Source: CAD feature listing. Evaluate the final solid. Frame: model axes, mm. Face numbers are marked on the shaded views. A direction names the side the tool comes from. Give positions to 0.01 mm unless a question says otherwise; leave off trailing zeros. Order: outer loops, then holes, each group sorted by start corner. A loop starts at its lowest first (then second) coordinate and runs counter-clockwise, first axis right, second up. Notation, with made-up numbers: (27.5, 36) -> (43.5, 36) arc R11 ccw to (43.5, 47) -> close; hole circle Ø4 at (72, 30). An arc over 180 degrees is marked (long way). Use one line per item in the form item = value. Start each with the question number.
from build123d import *

# Parameters (mm, degrees)
F0_R      = 76.2
F1_DEPTH  = 25.4
F2_R      = 5.08
F1_FACE_R = 71.12
F3_DEPTH  = 6.35
F4_R      = 3.175
F5_DEPTH  = 25.4
F6_R      = 59.059026
F7_DEPTH  = 21.59
F9_DEPTH  = 22.86
F11_DEPTH = 23.368
F13_DEPTH = 25.4


with BuildPart() as f1:
    # F0 (on Front) → F1 (new body)
    with BuildSketch(Plane.XZ):
        Circle(F0_R)
    extrude(amount=F1_DEPTH)

    # F2
    f2_edges = [f1.edges().sort_by_distance(p)[0] for p in [
        (76.2, -12.7, 0),
        (-76.2, 0, 0),
        (-76.2, -25.4, 0),
    ]]
    fillet(f2_edges, radius=F2_R)

    # F1_face (on face) → F3 (cut)
    with BuildSketch(Plane.XZ.offset(25.4)):
        Circle(F1_FACE_R)
    extrude(amount=-F3_DEPTH, mode=Mode.SUBTRACT)

    # F4 (on Front) → F5 (cut)
    with BuildSketch(Plane.XZ):
        with Locations((0, 66.04)):
            Circle(F4_R)
    extrude(amount=F5_DEPTH, mode=Mode.SUBTRACT)

    # F6 (on Front) → F7 (join)
    with BuildSketch(Plane.XZ):
        Circle(F6_R)
    extrude(amount=F7_DEPTH)

    # F8 (on Front) → F9 (join)
    with BuildSketch(Plane.XZ):
        Polygon((29.037268, -50.146991), (57.947202, 0.073516), (28.909934, 50.220507), (-29.037268, 50.146991), (-57.947202, -0.073516), (-28.909934, -50.220507), align=None)
    extrude(amount=F9_DEPTH)

    # F10 (on Front) → F11 (join)
    with BuildSketch(Plane.XZ):
        Polygon((-41.918568, 24.201697), (0, -48.403393), (41.918568, 24.201697), align=None)
    extrude(amount=F11_DEPTH)

    # F12 (on Front) → F13 (join)
    with BuildSketch(Plane.XZ):
        Polygon((33.022074, -0.404168), (28.800039, 16.161017), (16.861057, 28.395871), (0.404168, 33.022074), (-16.161017, 28.800039), (-28.395871, 16.861057), (-33.022074, 0.404168), (-28.800039, -16.161017), (-16.861057, -28.395871), (-0.404168, -33.022074), (16.161017, -28.800039), (28.395871, -16.861057), align=None)
    extrude(amount=F13_DEPTH)


solid = f1.part
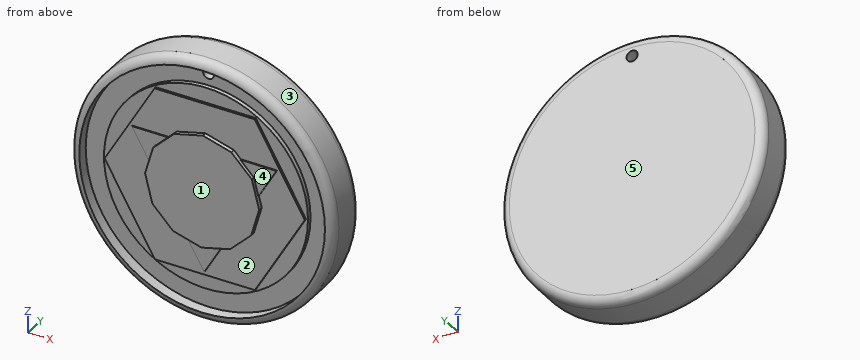
1) Pin query (flat end, axial travel): pin 1 (12 mm diameter, centred on x = -15, y = -4.5, fed in from +Z); pin 2 (12 mm diameter, centred on x = -59.5, y = -5.5, fed in from -Z); pin 3 (1 mm diameter, centred on y = -21.5, z = 27, fed in from -X). Return the tip coordinate at first contact, or that it passes through.
2) Reachability of the marked faces 4 and 5 from +Z, -Z, +X, -X, +Y, -Y: full face, straight path, thin tool, end or side. Return the list, or none.
3) Draft query along Z for the marked faces 1, 2 and 3. Return one class per face: +Z half, -Z half, draft (parallel to the pull), parting line (faces both ways), or undercut.
4) Cut plane A-A, the plane y = -9. Return the cut outline in (x, z) (3 decimals), plus the area to 3 significant figures.
5) Material intervals for probe 1 along Z at (x, y) = (0, -20.5); probe 2 along X at (y, z) = (-21.5, 21); probe 3 along Z at (x, y) = (43.5, -22.5), sorted ascending.
Output values:
q1.pin_1 = 75.66
q1.pin_2 = -54.26
q1.pin_3 = -71.33
q2.face_4 = -Y
q2.face_5 = +Z, -Z, +X, -X, +Y
q3.face_1 = draft
q3.face_2 = undercut
q3.face_3 = parting line
q4.outline = circle Ø152.4 at (0, 0); hole circle Ø6.35 at (0, 66.04)
q4.area = 18,200 mm^2
q5.probe_1 = -76.2 to -71.12, -59.06 to 59.06, 71.12 to 76.2
q5.probe_2 = -73.1 to -67.95, -55.2 to 55.2, 67.95 to 73.1
q5.probe_3 = -61.96 to -56.27, -25.02 to 25.02, 56.27 to 61.96
